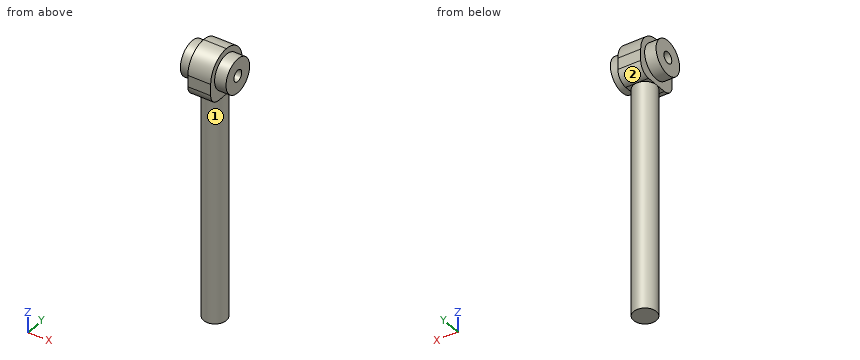
```python
from build123d import *

# Parameters (mm, degrees)
F0_R          = 6.35
F1_DEPTH      = 127
F2_W          = 12.7
F2_H          = 25.4
F3_DEPTH      = 25.4
F4_R          = 9.525
F4_R_2        = 3.175
F5_DEPTH      = 6.35
F5_DEPTH_BACK = 19.05
F6_DEPTH      = 25.4
F7_R          = 6.34999
F8_R          = 12.69999


# Not quite as in the source:
# - a fillet or chamfer is up to 0.001 mm smaller than in the source, because OpenCascade refuses the exact size


with BuildPart() as f1:
    # F0 (on Top) → F1 (new body)
    with BuildSketch(Plane.XY):
        Circle(F0_R)
    extrude(amount=F1_DEPTH)

    # F2 (on face) → F3 (join)
    with BuildSketch(Plane.XY.offset(127)):
        Rectangle(F2_W, F2_H)
    extrude(amount=F3_DEPTH)

    # F4 (on face) → F5 (join, two sides)
    with BuildSketch(Plane.YZ.offset(6.35)) as f5_sk:
        with Locations((0, 139.7)):
            Circle(F4_R)
        with Locations((0, 139.7)):
            Circle(F4_R_2, mode=Mode.SUBTRACT)
    extrude(amount=F5_DEPTH)
    extrude(f5_sk.sketch, amount=-F5_DEPTH_BACK)

    # F6 (cut): a face of the model
    f6_faces = [f1.faces().sort_by_distance(p)[0] for p in [
        (6.35, 0, 139.7),
    ]]
    extrude(f6_faces, amount=-F6_DEPTH, mode=Mode.SUBTRACT)

    # F7 (radius 6.35 in the source; OpenCascade refuses exactly that, so slightly less here)
    f7_edges = [f1.edges().sort_by_distance(p)[0] for p in [
        (0, -12.7, 127),
        (0, 12.7, 127),
    ]]
    fillet(f7_edges, radius=F7_R)

    # F8 (radius 12.7 in the source; OpenCascade refuses exactly that, so slightly less here)
    f8_edges = [f1.edges().sort_by_distance(p)[0] for p in [
        (0, -12.7, 152.4),
        (0, 12.7, 152.4),
    ]]
    fillet(f8_edges, radius=F8_R)


solid = f1.part
```
Model file for the job. Use its own axes, mm. Face numbers are marked on the shaded views. A direction names the side the tool comes from. Give positions to 0.01 mm unless a question says otherwise; leave off trailing zeros. Loops run counter-clockwise (first coordinate to the right, second up) from the corner with the lowest first, then second, coordinate; pieces in that order, holes last. Notation, with made-up numbers: (37, -17.75) - (58, -17.75) arc R21 cw to (58, 2.25) - close; hole circle Ø4 at (-19, 39). An arc over 180 degrees is marked (long way). One line per item, written item: value. Start each with the question number.
1. Pin check, flat tips, straight feed: pin 1 (5 mm diameter, centred on y = 1, z = 16.5, fed in from +X); pin 2 (2 mm diameter, centred on x = 1, z = 99.5, fed in from +Y); pin 3 (5.5 mm diameter, centred on y = 0, z = 139.7, fed in from -X); pin 4 (1 mm diameter, centred on x = -9.5, y = -4.5, fed in from -Z). Stop position of each tip, or through.
2. Which spindle directions (+Z, -Z, +X, -X, +Y, -Y) get a long thin tool onto all of the face, cutting with end or side? Do the marked faces 1 and 2. Say none if no direction does.
3. Slice it at B-B (z = 113). List the corners of the cut face in (x, y).
4. Probe L1, parallel to Z at x = 2.25, y = 0 (3 decimals); L2, parallel to Z at x = -9, y = 0 (3 decimals); L3, parallel to Y at x = 3, z = 139.7 (3 decimals). List the from-to ranges inside material, lowest first. Write a range as from..to.
5. Slice it at C-C (x = -9.5). List the corners of the cut face in (y, z) (3 decimals), plus the area to 3 significant figures.
Solution:
1. pin 1: stops at x = 6.35
1. pin 2: stops at y = 6.35
1. pin 3: passes through
1. pin 4: stops at z = 131.06
2. face 1: -Z
2. face 2: -Z, +X, -X, +Y
3. outline: circle Ø12.7 at (0, 0)
4. L1: z = 0..136.525, 142.875..152.4
4. L2: z = 130.175..136.525, 142.875..149.225
4. L3: y = -12.7..-3.175, 3.175..12.7
5. outline: circle Ø19.05 at (0, 139.7); hole circle Ø6.35 at (0, 139.7)
5. area: 253 mm^2
